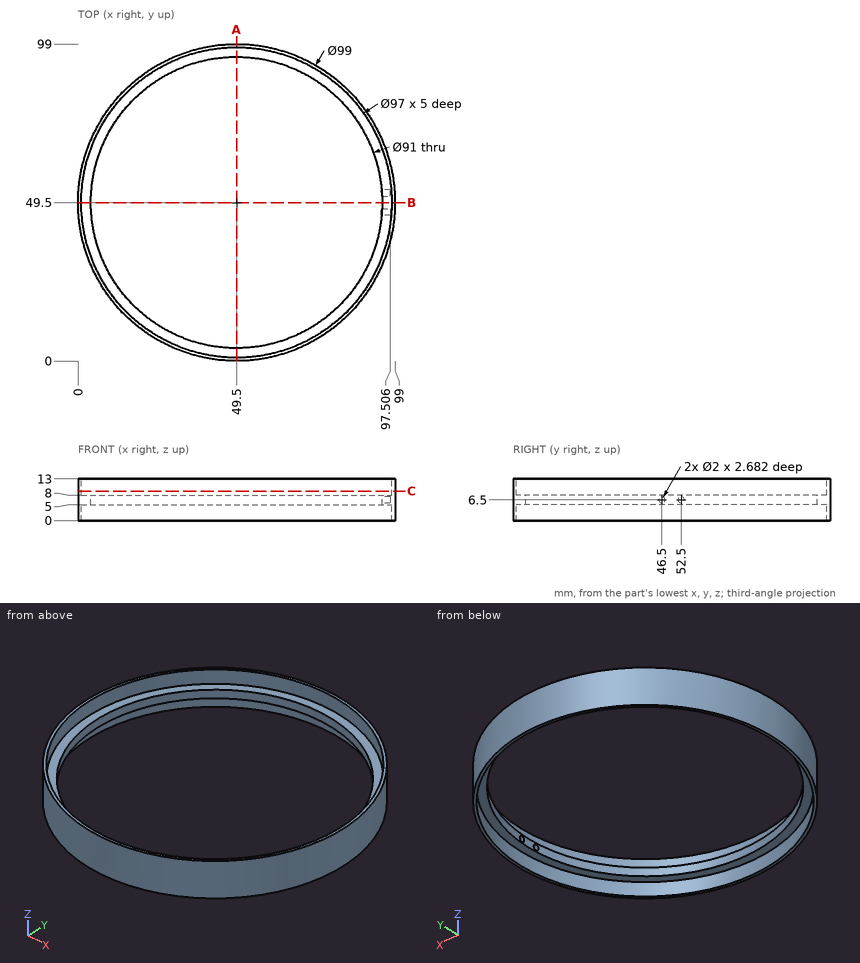
For this review, use the dimensioned drawing (mm, ordinates from the lowest corner) and the shaded views. Coordinates: 2 decimals unless noted, no trailing zeros. Loops run counter-clockwise (first coordinate to the right, second up) from the corner with the lowest first, then second, coordinate; pieces in that order, holes last. Notation, with made-up numbers: (8, 63.5) -> (36, 63.5) arc R21 ccw to (36, 79.5) -> close; hole circle Ø7 at (88.25, 52). An arc over 180 degrees is marked (long way). Use a Markdown table: item, result. Add a question column.
Item 1: Wall thickness on L1, parallel to Z at x = 96.9, y = 46.5; L2, parallel to Y at x = 49.5, z = 9.4; L3, parallel to Y at x = 49.5, z = 5.75: over which ranges is each line inside the solid? List them lowest first. Write a range as from..to.
Item 2: We need section C-C, the plane z = 9.25. Write out the cut boundary in (x, y).
Item 3: Clearance check with flat-ended pins moving along their axes: P1, Ø1.8, axis at y = 46.5, z = 6.5, coming from the -X side; P2, Ø6, axis at x = 32.5, z = 9, coming from the +Y side; P3, Ø2.5, axis at y = 52.5, z = 6.5, coming from the +X side. State where each tip first meets the part, or that it passes through.
Item 4: We need section A-A, the plane x = 49.5. Write out the cut boundary in (y, z), and give its area (3 significant figures).
Numbers:
| question | item | result |
|---|---|---|
| 1 | L1 | z = 5..5.5, 7.5..8 |
| 1 | L2 | y = 0..1, 98..99 |
| 1 | L3 | y = 0..4, 95..99 |
| 2 | outline | circle Ø99 at (49.5, 49.5); hole circle Ø97 at (49.5, 49.5) |
| 3 | P1 | stops at x = 0.04 |
| 3 | P2 | stops at y = 96.98 |
| 3 | P3 | stops at x = 98.97 |
| 4 | outline | (0, 0) -> (1, 0) -> (1, 5) -> (4, 5) -> (4, 8) -> (1, 8) -> (1, 13) -> (0, 13) -> close; (95, 5) -> (98, 5) -> (98, 0) -> (99, 0) -> (99, 13) -> (98, 13) -> (98, 8) -> (95, 8) -> close |
| 4 | area | 44.0 mm^2 |
